Geometry: see drawing. Coordinates: mm, zero at the bounding-box minimum. A direction names the side the tool comes from. Give positions to 0.01 mm unless a question says otherwise; leave off trailing zeros. Loops run counter-clockwise (first coordinate to the right, second up) from the corner with the lowest first, then second, coordinate; pieces in that order, holes last. Notation, with made-up numbers: (29.5, 54.5) -> (82.5, 54.5) arc R27 ccw to (82.5, 73.5) -> close; hole circle Ø2 at (-31, 68). An arc over 180 degrees is marked (long way). Return JSON: item names as keys, results as strings. Group by question number.
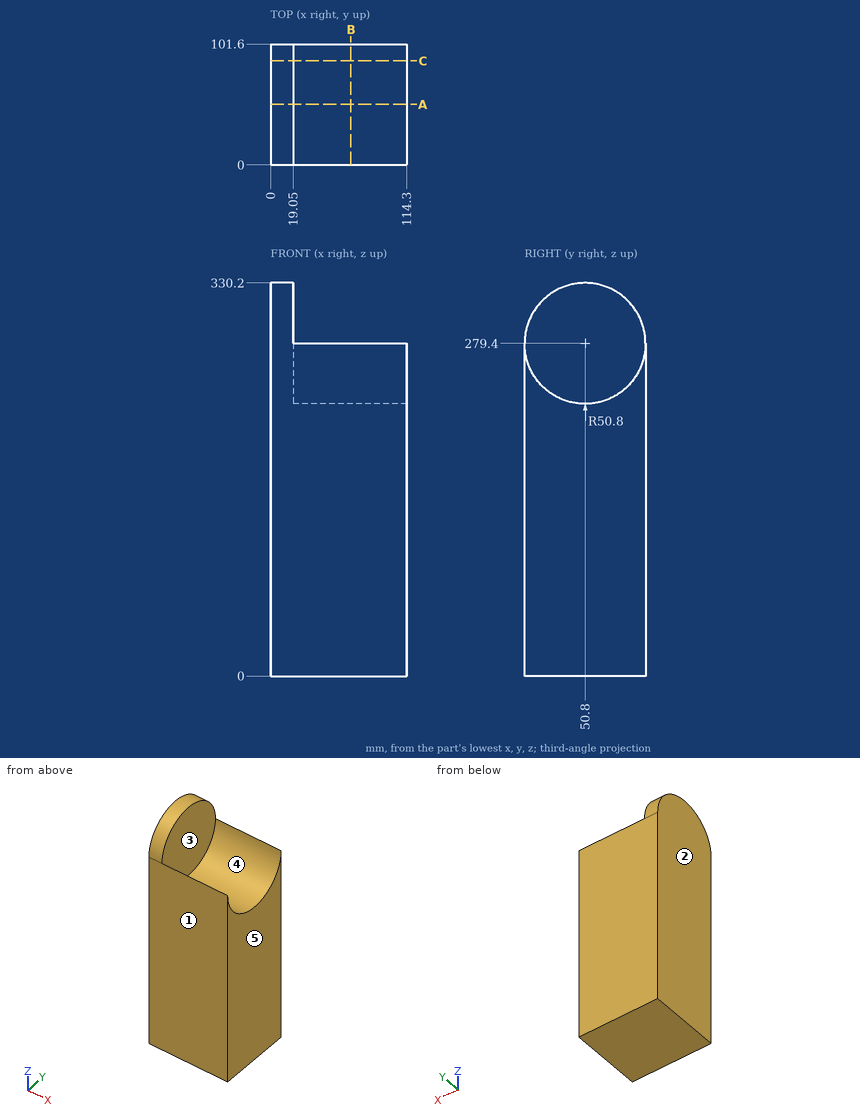
1) Contact query for a flat-ended pin moving along its axis: P1, Ø8, axis at x = 25, z = 292, coming from the -Y side. Output: stop coordinate, or through.
2) Cut plane B-B on x = 67.5. Return loops of the section in (y, z).
3) Cut plane C-C on y = 87.5. Return loops of the section in (x, z).
4) Material intervals for line 1 (X direction, y = 82.5, z = 283.5); line 2 (Y direction, x = 53.5, z = 239.5); line 3 (Z direction, x = 22, y = 87), sorted ascending.
5) Mould query, pull axis Y, two halves, no side actions, for the marked faces 1, 2 and 3. Classes: released by +Y, released by -Y, zero draft, split by the parting line, or undercut.
6) Reachability of the marked faces 4 and 5 from +Z, -Z, +X, -X, +Y, -Y: full face, straight path, thin tool, end or side. Return the list, or none.
7) Cut plane A-A on y = 50.8. Return loops of the section in (x, z).
Calculated:
{
 "1": {"P1": "through"},
 "2": {"outline": "(0, 0) -> (101.6, 0) -> (101.6, 279.4) arc R50.8 cw to (0, 279.4) -> close"},
 "3": {"outline": "(0, 0) -> (114.3, 0) -> (114.3, 244.28) -> (19.05, 244.28) -> (19.05, 314.52) -> (0, 314.52) -> close"},
 "4": {"line 1": "0 to 19.05", "line 2": "0 to 19.36, 82.24 to 101.6", "line 3": "0 to 243.76"},
 "5": {"face 1": "released by -Y", "face 2": "zero draft", "face 3": "undercut"},
 "6": {"face 4": "+Z, +X", "face 5": "+Z, -Z, +X, +Y, -Y"},
 "7": {"outline": "(0, 0) -> (114.3, 0) -> (114.3, 228.6) -> (19.05, 228.6) -> (19.05, 330.2) -> (0, 330.2) -> close"}
}
